from build123d import *

# Parameters (mm, degrees)
SKETCH1_W           = 32.766
SKETCH1_H           = 26.924
BOSS_EXTRUDE1_DEPTH = 27.686
BOSS_EXTRUDE2_DEPTH = 2.032
BOSS_EXTRUDE3_DEPTH = 2.032


with BuildPart() as part:
    # Sketch1 → Boss-Extrude1 (new body)
    with BuildSketch(Plane(origin=(0, 0, 0), x_dir=(1, 0, 0), z_dir=(0, 1, 0))):
        with Locations((-1.646230698, -0.06385993)):
            Rectangle(SKETCH1_W, SKETCH1_H)
    extrude(amount=BOSS_EXTRUDE1_DEPTH)

    # Sketch1<12> → Boss-Extrude2 (add)
    with BuildSketch(Plane(origin=(0, 0, 0), x_dir=(1, 0, 0), z_dir=(0, 1, 0))):
        with BuildLine():
            Line((-18.029230698, 13.39814007), (-18.029230698, -13.52585993))
            Line((-18.029230698, -13.52585993), (-24.125230698, -13.52585993))
            Line((-24.125230698, -13.52585993), (-26.411230698, -11.23985993))
            Line((-26.411230698, -11.23985993), (-26.411230698, -1.71485993))
            Line((-26.411230698, -1.71485993), (-23.109230698, -1.71485993))
            ThreePointArc((-23.109230698, -1.71485993), (-21.458230698, -0.06385993), (-23.109230698, 1.58714007))
            Line((-23.109230698, 1.58714007), (-26.411230698, 1.58714007))
            Line((-26.411230698, 1.58714007), (-26.411230698, 11.11214007))
            Line((-26.411230698, 11.11214007), (-24.125230698, 13.39814007))
            Line((-24.125230698, 13.39814007), (-18.029230698, 13.39814007))
        make_face()
    extrude(amount=BOSS_EXTRUDE2_DEPTH)

    # Sketch1<13> → Boss-Extrude3 (add)
    with BuildSketch(Plane(origin=(0, 0, 0), x_dir=(1, 0, 0), z_dir=(0, 1, 0))):
        with BuildLine():
            Line((20.832769302, -13.52585993), (14.736769302, -13.52585993))
            Line((14.736769302, -13.52585993), (14.736769302, 13.39814007))
            Line((14.736769302, 13.39814007), (20.832769302, 13.39814007))
            Line((20.832769302, 13.39814007), (23.118769302, 11.11214007))
            Line((23.118769302, 11.11214007), (23.118769302, 1.58714007))
            Line((23.118769302, 1.58714007), (19.816769302, 1.58714007))
            ThreePointArc((19.816769302, 1.58714007), (18.165769302, -0.06385993), (19.816769302, -1.71485993))
            Line((19.816769302, -1.71485993), (23.118769302, -1.71485993))
            Line((23.118769302, -1.71485993), (23.118769302, -11.23985993))
            Line((23.118769302, -11.23985993), (20.832769302, -13.52585993))
        make_face()
    extrude(amount=BOSS_EXTRUDE3_DEPTH)


solid = part.part
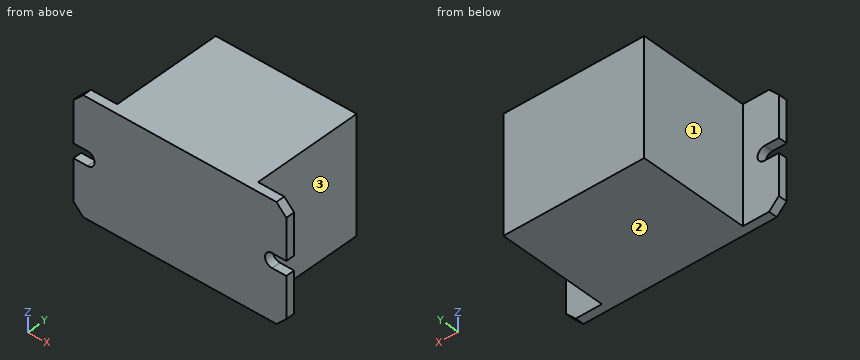
Geometry check sheet. Reference: the model listing, model coordinates, mm. Face numbers are marked on the shaded views. A direction names the side the tool comes from. Give positions to 0.01 mm unless a question says otherwise; leave off trailing zeros. Write each loop counter-clockwise with the first axis right and the second up, starting at its lowest first coordinate (ties: lowest second). Pieces come first, ordered by that corner, then holes. Notation, with made-up numbers: M 15,-2 L 71,-2 A13 ccw 71,20 Z; hole C 67.5,16 d11. An arc over 180 degrees is marked long. One line per question, with ' | ' between items.
1. Cross-section at D-D (z = 1). Enter the section's corners in (x, y).
Ans:
outline: M -21.75,0 L 18.46,0 L 18.46,2.03 L 14.74,2.03 L 14.74,27.69 L -18.03,27.69 L -18.03,2.03 L -21.75,2.03 Z
2. Scan lines: line 1 along X through (y, z) = (21, -8); line 2 along Y through (x, z) = (-20, 3.5). Record each from-to range of solid material in increasing order. Write a range as from..to.
Ans:
line 1: -18.03..14.74 | line 2: 0..2.03
3. Cross-section at C-C (y = 9.5). Enter the section's corners in (x, z).
Ans:
outline: M -18.03,-13.4 L 14.74,-13.4 L 14.74,13.53 L -18.03,13.53 Z
4. Gauge pin test, flat ends, axial feed: pin 1 (1 mm diameter, centred on y = 10.5, z = 10, fed in from +X); pin 2 (6 mm diameter, centred on y = 20.5, z = -5.5, fed in from -X); pin 3 (6.5 mm diameter, centred on x = 20.5, z = 1.5, fed in from +Y). Record the tip position at first contact, or that the pin passes through.
Ans:
pin 1: x = 14.74 | pin 2: x = -18.03 | pin 3: y = 2.03
5. Set-up check for the marked faces 1, 2 and 3: record each of +Z, -Z, +X, -X, +Y, -Y from which the full face is reachable in a straight line by a thin tool's end or side.
Ans:
face 1: +Z, -Z, -X, +Y | face 2: -Z, +X, -X, +Y, -Y | face 3: +Z, -Z, +X, +Y
6. Cross-section at A-A (x = 19). Enter the section's corners in (y, z).
Ans:
outline: M 0,-13.4 L 2.03,-13.4 L 2.03,-1.37 L 0,-1.37 Z; M 0,1.5 L 2.03,1.5 L 2.03,13.53 L 0,13.53 Z
7. Cross-section at B-B (z = -5.75). Enter the section's corners in (x, y), plus the area to 3 significant figures.
Ans:
outline: M -26.41,0 L 23.12,0 L 23.12,2.03 L 14.74,2.03 L 14.74,27.69 L -18.03,27.69 L -18.03,2.03 L -26.41,2.03 Z | area: 941 mm2
